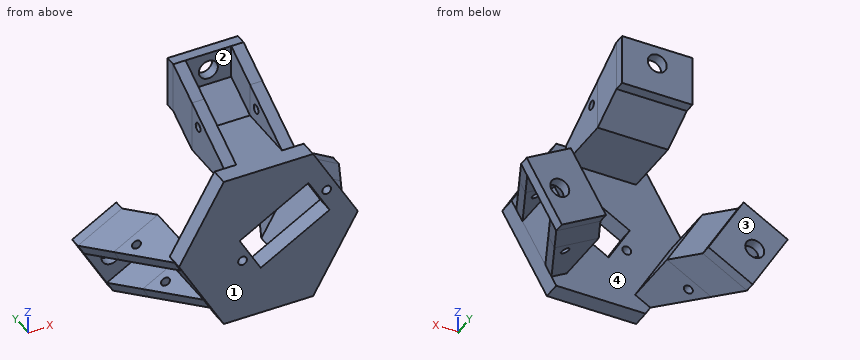
```python
from build123d import *

# Parameters (mm, degrees)
BOSS_EXTRUDE1_DEPTH         = 5
SKETCH4_W                   = 20
SKETCH4_H                   = 5
BOSS_EXTRUDE3_DEPTH         = 17
BOSS_EXTRUDE2_START         = 6.5
SKETCH2_R                   = 1.25
BOSS_EXTRUDE2_DEPTH         = 3.5
CIRPATTERN1_COUNT           = 3
CIRPATTERN1_COPY_1_SKETCH_W = 20
CIRPATTERN1_COPY_1_SKETCH_H = 5
CIRPATTERN1_COPY_1_DEPTH    = 17
CIRPATTERN1_COPY_2_SKETCH_W = 20
CIRPATTERN1_COPY_2_SKETCH_H = 5
CIRPATTERN1_COPY_2_DEPTH    = 17
CIRPATTERN1_START           = 6.5
CIRPATTERN1_COPY_3_SKETCH_R = 1.25
CIRPATTERN1_COPY_3_DEPTH    = 3.5
CIRPATTERN1_COPY_4_SKETCH_R = 1.25
CIRPATTERN1_COPY_4_DEPTH    = 3.5
CUT_EXTRUDE1_REACH          = 50.2
CUT_EXTRUDE2_REACH          = 50.2
SKETCH6_R                   = 1.25
BOSS_EXTRUDE4_DEPTH         = 3
CUT_EXTRUDE3_REACH          = 61.959
SKETCH13_R                  = 2.7
CIRPATTERN2_COUNT           = 3


with BuildPart() as part:
    # Sketch1 → Boss-Extrude1 (new body)
    with BuildSketch(Plane(origin=(0, 0, 0), x_dir=(1, 0, 0), z_dir=(0, 1, 0))):
        Polygon((25.403411844, 0), (12.701705922, 22), (-12.701705922, 22), (-25.403411844, 0), (-12.701705922, -22), (12.701705922, -22), align=None)
    extrude(amount=BOSS_EXTRUDE1_DEPTH)

    # Sketch4 → Boss-Extrude3 (add)
    with BuildSketch(Plane(origin=(0, 5, 0), x_dir=(1, 0, 0), z_dir=(0, 1, 0))):
        with Locations((0, -19.5)):
            Rectangle(SKETCH4_W, SKETCH4_H)
    boss_extrude3 = extrude(amount=BOSS_EXTRUDE3_DEPTH)

    # Sketch2 → Boss-Extrude2 (add)
    with BuildSketch(Plane(origin=(0, 0, 0), x_dir=(0, 0, -1), z_dir=(1, 0, 0)).offset(BOSS_EXTRUDE2_START)):
        Polygon((-22, 22), (-22, 5), (-31.5, 22), align=None)
        with Locations(Location((-26, 18.75, 0), (0, 0, 180))):
            Circle(SKETCH2_R, mode=Mode.SUBTRACT)
    boss_extrude2 = extrude(amount=BOSS_EXTRUDE2_DEPTH)

    # Mirror1: Boss-Extrude3, Boss-Extrude2 across plane
    add(boss_extrude3.mirror(Plane(origin=(0, 0, 0), x_dir=(0, 0, 1), z_dir=(1, 0, 0))))
    add(boss_extrude2.mirror(Plane(origin=(0, 0, 0), x_dir=(0, 0, 1), z_dir=(1, 0, 0))))

    # CirPattern1: Boss-Extrude3, Boss-Extrude2 ×3 about axis
    cirpattern1_axis = Axis((0, 0, 0), (0, 1, 0))
    add([boss_extrude3.rotate(cirpattern1_axis, i * 360 / CIRPATTERN1_COUNT) for i in range(1, CIRPATTERN1_COUNT)])
    add([boss_extrude2.rotate(cirpattern1_axis, i * 360 / CIRPATTERN1_COUNT) for i in range(1, CIRPATTERN1_COUNT)])

    # CirPattern1 copy 1 sketch → CirPattern1 copy 1 (add)
    with BuildSketch(Plane(origin=(0, 5, 0), x_dir=(0.4999999999999998, 0, 0.8660254037844387), z_dir=(0, 1, 0))):
        with Locations((0, 19.5)):
            Rectangle(CIRPATTERN1_COPY_1_SKETCH_W, CIRPATTERN1_COPY_1_SKETCH_H)
    extrude(amount=CIRPATTERN1_COPY_1_DEPTH)

    # CirPattern1 copy 2 sketch → CirPattern1 copy 2 (add)
    with BuildSketch(Plane(origin=(0, 5, 0), x_dir=(0.5000000000000004, 0, -0.8660254037844384), z_dir=(0, 1, 0))):
        with Locations((0, 19.5)):
            Rectangle(CIRPATTERN1_COPY_2_SKETCH_W, CIRPATTERN1_COPY_2_SKETCH_H)
    extrude(amount=CIRPATTERN1_COPY_2_DEPTH)

    # CirPattern1 copy 3 sketch → CirPattern1 copy 3 (add)
    with BuildSketch(Plane(origin=(0, 0, 0), x_dir=(-0.8660254037844387, 0, 0.4999999999999998), z_dir=(0.4999999999999998, 0, 0.8660254037844387)).offset(CIRPATTERN1_START)):
        Polygon((-22, -22), (-22, -5), (-31.5, -22), align=None)
        with Locations((-26, -18.75)):
            Circle(CIRPATTERN1_COPY_3_SKETCH_R, mode=Mode.SUBTRACT)
    extrude(amount=CIRPATTERN1_COPY_3_DEPTH)

    # CirPattern1 copy 4 sketch → CirPattern1 copy 4 (add)
    with BuildSketch(Plane(origin=(0, 0, 0), x_dir=(0.8660254037844384, 0, 0.5000000000000004), z_dir=(0.5000000000000004, 0, -0.8660254037844384)).offset(CIRPATTERN1_START)):
        Polygon((-22, -22), (-22, -5), (-31.5, -22), align=None)
        with Locations((-26, -18.75)):
            Circle(CIRPATTERN1_COPY_4_SKETCH_R, mode=Mode.SUBTRACT)
    extrude(amount=CIRPATTERN1_COPY_4_DEPTH)

    # Sketch3 → Cut-Extrude1 (cut, up to next)
    with BuildSketch(Plane(origin=(0, 5, 0), x_dir=(1, 0, 0), z_dir=(0, 1, 0)), mode=Mode.PRIVATE) as cut_extrude1_sk1:
        Polygon((-2.196152423, 8.196152423), (17.376021703, -3.103847577), (11.376021703, -13.496152423), (-8.196152423, -2.196152423), align=None)
    cut_extrude1_tool1 = extrude(cut_extrude1_sk1.sketch, amount=-CUT_EXTRUDE1_REACH, mode=Mode.PRIVATE) & part.part
    add(cut_extrude1_tool1.solids().sort_by_distance((4.589935, 5, 2.65))[0], mode=Mode.SUBTRACT)

    # Sketch6 → Cut-Extrude2 (cut, up to next)
    with BuildSketch(Plane(origin=(0, 5, 0), x_dir=(1, 0, 0), z_dir=(0, 1, 0)), mode=Mode.PRIVATE) as cut_extrude2_sk1:
        with Locations(Location((-7.361215932, 4.25, 0), (0, 0, 270))):
            Circle(SKETCH6_R)
    cut_extrude2_tool1 = extrude(cut_extrude2_sk1.sketch, amount=-CUT_EXTRUDE2_REACH, mode=Mode.PRIVATE) & part.part
    # Sketch6 → Cut-Extrude2 (cut, up to next)
    with BuildSketch(Plane(origin=(0, 5, 0), x_dir=(1, 0, 0), z_dir=(0, 1, 0)), mode=Mode.PRIVATE) as cut_extrude2_sk2:
        with Locations(Location((16.541085212, -9.55, 0), (0, 0, 270))):
            Circle(SKETCH6_R)
    cut_extrude2_tool2 = extrude(cut_extrude2_sk2.sketch, amount=-CUT_EXTRUDE2_REACH, mode=Mode.PRIVATE) & part.part
    add(cut_extrude2_tool1.solids().sort_by_distance((-7.361216, 5, -4.25))[0], mode=Mode.SUBTRACT)
    add(cut_extrude2_tool2.solids().sort_by_distance((16.541085, 5, 9.55))[0], mode=Mode.SUBTRACT)

    # Sweep1: sweep along a path in Sketch11
    with BuildLine(Plane(origin=(-5, 0, 8.660254038), x_dir=(0.8660254037844364, 0, 0.5000000000000041), z_dir=(-0.500000000000004, 0, 0.8660254037844363))) as sweep1_path:
        Line((-31.5, 22), (-37.088235294, 32))
    # Sketch10 → Sweep1 (sweep)
    with BuildSketch(Plane(origin=(0, 22, 0), x_dir=(1, 0, 0), z_dir=(0, 1, 0))):
        Polygon((-22.279800219, 24.410254038), (-9.722431864, 17.160254038), (-19.722431864, -0.160254038), (-32.279800219, 7.089745962), (-30.529800219, 10.120834875), (-22.302558883, 5.370834875), (-15.802558883, 16.629165125), (-24.029800219, 21.379165125), align=None)
    sweep1 = sweep(path=sweep1_path.line)

    # Sketch12 → Boss-Extrude4 (add)
    with BuildSketch(Plane(origin=(0, 32, 0), x_dir=(1, 0, 0), z_dir=(0, 1, 0))):
        Polygon((-27.119353946, 27.204371685), (-14.561985591, 19.954371685), (-24.561985591, 2.633863609), (-37.119353946, 9.883863609), align=None)
    boss_extrude4 = extrude(amount=BOSS_EXTRUDE4_DEPTH)

    # Sketch13 → Cut-Extrude3 (cut, up to next)
    with BuildSketch(Plane(origin=(0, 35, 0), x_dir=(1, 0, 0), z_dir=(0, 1, 0)), mode=Mode.PRIVATE) as cut_extrude3_sk1:
        with Locations(Location((-27.712812921, 16, 0), (0, 0, 270))):
            Circle(SKETCH13_R)
    cut_extrude3_tool1 = extrude(cut_extrude3_sk1.sketch, amount=-CUT_EXTRUDE3_REACH, mode=Mode.PRIVATE) & part.part
    cut_extrude3 = cut_extrude3_tool1.solids().sort_by_distance((-27.712813, 35, -16))[0]
    add(cut_extrude3, mode=Mode.SUBTRACT)

    # CirPattern2: Sweep1, Boss-Extrude4, Cut-Extrude3 ×3 about axis
    cirpattern2_axis = Axis((0, 0, 0), (0, 1, 0))
    add([sweep1.rotate(cirpattern2_axis, i * 360 / CIRPATTERN2_COUNT) for i in range(1, CIRPATTERN2_COUNT)])
    add([boss_extrude4.rotate(cirpattern2_axis, i * 360 / CIRPATTERN2_COUNT) for i in range(1, CIRPATTERN2_COUNT)])
    add([cut_extrude3.rotate(cirpattern2_axis, i * 360 / CIRPATTERN2_COUNT) for i in range(1, CIRPATTERN2_COUNT)], mode=Mode.SUBTRACT)


solid = part.part
```
Geometry check sheet. Reference: the model listing, model coordinates, mm. Face numbers are marked on the shaded views. A direction names the side the tool comes from. Give positions to 0.01 mm unless a question says otherwise; leave off trailing zeros. Write each loop counter-clockwise with the first axis right and the second up, starting at its lowest first coordinate (ties: lowest second). Pieces come first, ordered by that corner, then holes. Notation, with made-up numbers: (-34.5, 33.25) -> (6.5, 33.25) arc R33 cw to (6.5, 65.25) -> close; hole circle Ø6 at (63.5, 78.25). An arc over 180 degrees is marked (long way). Use one line per item in the form item = value.
Item 1: Sectioned sample at D-D on z = -12. Enter the section's corners in (x, y), plus the area to 3 significant figures.
Results list:
outline = (-35.9, 32) -> (-33.78, 28.73) -> (-33.78, 32) -> (-24.93, 32) -> (-18.48, 22) -> (-18.48, 0) -> (18.48, 0) -> (18.48, 22) -> (24.93, 32) -> (33.78, 32) -> (33.78, 28.73) -> (35.9, 32) -> (35.9, 35) -> (19.15, 35) -> (19.15, 32) -> (12.7, 22) -> (12.7, 5) -> (-12.7, 5) -> (-12.7, 22) -> (-19.15, 32) -> (-19.15, 35) -> (-35.9, 35) -> close
area = 604 mm2
Item 2: Depth check by flat-ended pin: pin 1 Ø1.5 at (x, z) = (13, -10.5) entering from +Y; pin 2 Ø0.9 at (y, z) = (33, 26.5) entering from -X; pin 3 Ø5 at (x, y) = (26, 6) entering from +Z. Enter the tip coordinate at first touch or a pass-through.
Results list:
pin_1 = 22.46
pin_2 = -10
pin_3 = 2.94
Item 3: Access from +Z, -Z, +X, -X, +Y, -Y to the whole of each face (thin tool, end or side, straight path). Record for the marked faces 1 and 2.
Results list:
face_1 = +Z, -Z, +X, -X, -Y
face_2 = +Z, -Y
Item 4: Mould release check, pull along X, two halves, no side actions. Record for the marked faces 3 and 4: released by +X, released by -X, zero draft, split by the parting line, or undercut.
Results list:
face_3 = zero draft
face_4 = undercut
Item 5: Sectioned sample at A-A on y = 8.5. Enter the section's corners in (x, z), plus the area to 3 significant figures.
Results list:
outline = (-25.75, -3.32) -> (-24, -6.35) -> (-22.3, -5.37) -> (-15.8, -16.63) -> (-17.5, -17.61) -> (-15.75, -20.64) -> (-9.72, -17.16) -> (-19.72, 0.16) -> close; (-10, 17) -> (10, 17) -> (10, 23.96) -> (6.5, 23.96) -> (6.5, 22) -> (-6.5, 22) -> (-6.5, 23.96) -> (-10, 23.96) -> close; (9.72, -17.16) -> (15.75, -20.64) -> (17.5, -17.61) -> (15.8, -16.63) -> (22.3, -5.37) -> (24, -6.35) -> (25.75, -3.32) -> (19.72, 0.16) -> close
area = 341 mm2
Item 6: Sectioned sample at C-C on x = 0. Enter the section's corners in (y, z), plus the area to 3 significant figures.
Results list:
outline = (0, -22) -> (5, -22) -> (5, -6.93) -> (0, -6.93) -> close; (0, 6.93) -> (5, 6.93) -> (5, 17) -> (22, 17) -> (32, 22.59) -> (35, 22.59) -> (35, 29.3) -> (32, 29.3) -> (32, 27.59) -> (22, 22) -> (0, 22) -> close; (32, 34.7) -> (35, 34.7) -> (35, 37.09) -> (32, 37.09) -> close
area = 313 mm2
Item 7: Scan lines: line 1 (X direction, y = 20, z = 25); line 2 (X direction, y = 33, z = 32); line 3 (X direction, y = 34.2, z = -16). Record each from-to range of solid material in increasing order.
Results list:
line_1 = -10 to -6.5, 6.5 to 10
line_2 = -10 to -2.7, 2.7 to 10
line_3 = -33.59 to -30.41, -25.01 to -16.85, 16.85 to 25.01, 30.41 to 33.59
Item 8: Sectioned sample at B-B on z = 9.55. Enter the section's corners in (x, y), plus the area to 3 significant figures.
Results list:
outline = (-19.89, 0) -> (4.54, 0) -> (4.54, 5) -> (-19.89, 5) -> close; (13.65, 0) -> (15.29, 0) -> (15.29, 5) -> (13.65, 5) -> close; (17.79, 0) -> (19.89, 0) -> (19.89, 5) -> (17.79, 5) -> close
area = 141 mm2
